Check sheet for the modelled part. Datum: model origin and axes. Units: mm. Face numbers are marked on the shaded views. A direction names the side the tool comes from. Give positions to 0.01 mm unless a question says otherwise; leave off trailing zeros. Order: outer loops, then holes, each group sorted by start corner. A loop starts at its lowest first (then second) coordinate and runs counter-clockwise, first axis right, second up. Notation, with made-up numbers: (2.5, 36) -> (20.5, 36) arc R21 cw to (20.5, 75) -> close; hole circle Ø5 at (-9, 28). An arc over 180 degrees is marked (long way). Answer in a Markdown table with one row per item. Add a question column.
(1) Set-up check for the marked faces 4 and 5: record each of +Z, -Z, +X, -X, +Y, -Y from which the full face is reachable in a straight line by a thin tool's end or side.
(2) Cross-section at A-A (x = -21.2). Record the cut outline in (y, z).
(3) Cross-section at D-D (x = -9). Record the cut outline in (y, z), then the cut area to 3 significant figures.
(4) Thickness scan on L1, parallel to Y at x = 8, z = 1.9; L2, parallel to Y at x = -21.2, z = 1.55; L3, parallel to Y at x = -4, z = 2.95. Record the ranges inside material, lowest first. Write a range as [from, to].
(5) Cross-section at B-B (y = 7.5). Record the cut outline in (x, z).
(6) Cross-section at C-C (z = 1.5). State how many separate pieces and enclosed holes the cut face has, then the cut area to 3 significant figures.
(7) Go/stop test with flat-tipped pins: pin 1 (1.2 mm diameter, centred on x = 22.5, z = 2, fed in from -Y); pin 2 (0.9 mm diameter, centred on y = 10, z = 1.5, fed in from -X); pin 3 (1.5 mm diameter, centred on x = -14.5, y = 15.5, fed in from -Z); pin 4 (1 mm diameter, centred on y = 9, z = 1, fed in from +X). Record where each tip stops, or that it passes through.
(8) Release check for a two-part mould opening along Y. For the marked faces 1, 2 and 3 record: released by +Y, released by -Y, zero draft, split by the parting line, or undercut.
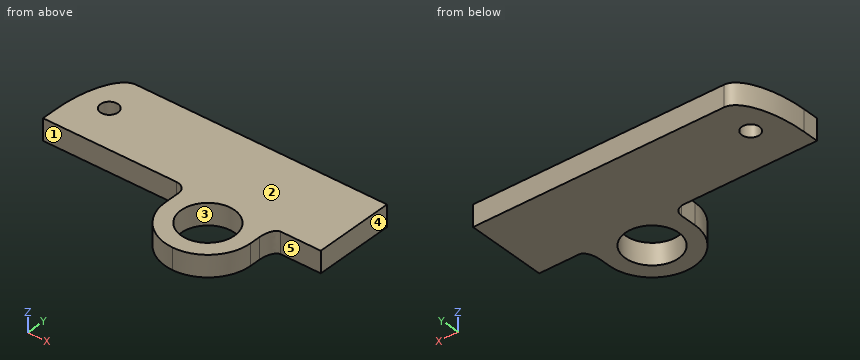
```python
from build123d import *

# Parameters (mm, degrees)
RESSALTO_EXTRUS_O1_DEPTH = 4
FILETE3_R                = 8
ESBO_O2_R                = 1.65
ESBO_O2_R_2              = 5
CORTE_EXTRUS_O1_DEPTH    = 40.102429592
FILETE12_SIZE            = 5
FILETE12_SIZE_2          = 12
FILETE14_R               = 2
ESBO_O3_W                = 9
ESBO_O3_H                = 13
CORTE_EXTRUS_O2_DEPTH    = 40.102429743
FILETE15_R               = 8
FILETE16_SIZE            = 3
FILETE16_SIZE_2          = 1.5


# Some blends are built 0.0001 mm under size
with BuildPart() as part:
    # Esboço1 → Ressalto-extrusão1 (new body)
    with BuildSketch(Plane.XY):
        Polygon((0, 0), (25, 0), (25, 28), (-27, 28), (-27, 13), (0, 13), align=None)
    extrude(amount=RESSALTO_EXTRUS_O1_DEPTH)

    # Filete3
    filete3_edges = [part.edges().sort_by_distance(p)[0] for p in [
        (0, 0, 2),
    ]]
    fillet(filete3_edges, radius=FILETE3_R)

    # Esboço2 → Corte-extrusão1 (cut, through all)
    with BuildSketch(Plane.XY.offset(4)):
        with Locations((-21.2, 21)):
            Circle(ESBO_O2_R)
        with Locations((8, 8)):
            Circle(ESBO_O2_R_2)
    extrude(amount=-CORTE_EXTRUS_O1_DEPTH, mode=Mode.SUBTRACT)

    # Filete12
    # an asymmetric fillet: 12, 5 mm, written as the material it takes off along each edge
    with BuildSketch(Plane(origin=(-27, 28, -30), x_dir=(1, 0, 0), z_dir=(0, 0, 1))) as filete12_piece_1:
        with BuildLine():
            Bezier((FILETE12_SIZE, 0), (0, 0), (0, -FILETE12_SIZE_2), weights=[1, 0.707106781, 1])
            Line((0, -FILETE12_SIZE_2), (0, 0))
            Line((0, 0), (FILETE12_SIZE, 0))
        make_face()
    extrude(amount=64, mode=Mode.SUBTRACT)

    # Filete14
    filete14_edges = [part.edges().sort_by_distance(p)[0] for p in [
        (0, 13, 2),
    ]]
    fillet(filete14_edges, radius=FILETE14_R)

    # Esboço3 → Corte-extrusão2 (cut, through all)
    with BuildSketch(Plane.XY.offset(4)):
        with Locations((20.5, 6.5)):
            Rectangle(ESBO_O3_W, ESBO_O3_H)
    extrude(amount=-CORTE_EXTRUS_O2_DEPTH, mode=Mode.SUBTRACT)

    # Filete15
    filete15_edges = [part.edges().sort_by_distance(p)[0] for p in [
        (16, 0, 2),
    ]]
    fillet(filete15_edges, radius=FILETE15_R - 0.0001)  # a hair under: the kernel refuses the full size

    # Filete16
    # an asymmetric fillet: 3, 1.5 mm, written as the material it adds along each edge
    with BuildSketch(Plane(origin=(16, 13, 4), x_dir=(0, -1, 0), z_dir=(0, 0, -1))) as filete16_piece_1:
        with BuildLine():
            Bezier((FILETE16_SIZE, 0), (0, 0), (0, -FILETE16_SIZE_2), weights=[1, 0.707106781, 1])
            Line((0, -FILETE16_SIZE_2), (0, 0))
            Line((0, 0), (FILETE16_SIZE, 0))
        make_face()
    extrude(amount=4)


solid = part.part
```
Answer below:
| question | item | result |
|---|---|---|
| 1 | face 4 | +Z, -Z, +X, +Y, -Y |
| 1 | face 5 | +Z, -Z, +X, -Y |
| 2 | outline | (13, 0) -> (19.35, 0) -> (19.35, 4) -> (13, 4) -> close; (22.65, 0) -> (28, 0) -> (28, 4) -> (22.65, 4) -> close |
| 3 | outline | (13, 0) -> (28, 0) -> (28, 4) -> (13, 4) -> close |
| 3 | area | 60.0 mm² |
| 4 | L1 | y = [0, 3], [13, 28] |
| 4 | L2 | y = [13, 19.35], [22.65, 28] |
| 4 | L3 | y = [13, 28] |
| 5 | outline | (0.02, 0) -> (3.03, 0) -> (3.03, 4) -> (0.02, 4) -> close; (12.97, 0) -> (15.98, 0) -> (15.98, 4) -> (12.97, 4) -> close |
| 6 | separate pieces | 1 |
| 6 | enclosed holes | 2 |
| 6 | area | 862 mm² |
| 7 | pin 1 | stops at y = 13 |
| 7 | pin 2 | stops at x = 0 |
| 7 | pin 3 | stops at z = 0 |
| 7 | pin 4 | stops at x = 16 |
| 8 | face 1 | released by -Y |
| 8 | face 2 | zero draft |
| 8 | face 3 | undercut |
